```python
from build123d import *

# Parameters (mm, degrees)
SKETCH1_W           = 243
SKETCH1_H           = 30
BOSS_EXTRUDE1_DEPTH = 70
SKETCH2_W           = 120
SKETCH2_H           = 10
CUT_EXTRUDE1_DEPTH  = 70
FILLET1_R           = 3
SKETCH3_R           = 3
CUT_EXTRUDE2_DEPTH  = 20
SKETCH4_R           = 11.000191916
SKETCH4_R_2         = 5.90738233
BOSS_EXTRUDE2_DEPTH = 39
SKETCH5_R           = 1.5
CUT_EXTRUDE3_DEPTH  = 20


with BuildPart() as part:
    # Sketch1 → Boss-Extrude1 (new body)
    with BuildSketch(Plane(origin=(0, 0, 0), x_dir=(1, 0, 0), z_dir=(0, 1, 0))):
        with Locations((-94.428984733, -7.936828819)):
            Rectangle(SKETCH1_W, SKETCH1_H)
    extrude(amount=BOSS_EXTRUDE1_DEPTH)

    # Sketch2 → Cut-Extrude1 (cut)
    with BuildSketch(Plane(origin=(0, 70, 0), x_dir=(1, 0, 0), z_dir=(0, 1, 0))):
        with Locations((-45.928984733, 2.063171181)):
            Rectangle(SKETCH2_W, SKETCH2_H)
    extrude(amount=-CUT_EXTRUDE1_DEPTH, mode=Mode.SUBTRACT)

    # Fillet1
    fillet1_edges = [part.edges().sort_by_distance(p)[0] for p in [
        (14.071015267, 35, -7.063171181),
        (14.071015267, 35, 2.936828819),
        (-105.928984733, 35, 2.936828819),
        (-105.928984733, 35, -7.063171181),
    ]]
    fillet(fillet1_edges, radius=FILLET1_R)

    # Sketch3 → Cut-Extrude2 (cut)
    with BuildSketch(Plane(origin=(0, 0, 0), x_dir=(-1, 0, 0), z_dir=(0, -1, 0))):
        with Locations(Location((51.298984733, -12.077870123, 0), (0, 0, 90))):
            Circle(SKETCH3_R)
        with Locations(Location((185.928984733, -2.936828819, 0), (0, 0, 90))):
            Circle(SKETCH3_R)
    extrude(amount=-CUT_EXTRUDE2_DEPTH, mode=Mode.SUBTRACT)

    # Sketch4 → Boss-Extrude2 (add)
    with BuildSketch(Plane(origin=(0, 0, 0), x_dir=(-1, 0, 0), z_dir=(0, -1, 0))):
        with Locations((188.57546064, -9.351449297)):
            Circle(SKETCH4_R)
        with Locations((51.298984733, -12.077870123)):
            Circle(SKETCH4_R_2)
    extrude(amount=-BOSS_EXTRUDE2_DEPTH)

    # Sketch5 → Cut-Extrude3 (cut)
    with BuildSketch(Plane(origin=(0, 0, 0), x_dir=(-1, 0, 0), z_dir=(0, -1, 0))):
        with Locations(Location((51.298984733, -12.936828819, 0), (0, 0, 90))):
            Circle(SKETCH5_R)
        with Locations(Location((185.928984733, -2.936828819, 0), (0, 0, 90))):
            Circle(SKETCH5_R)
    extrude(amount=-CUT_EXTRUDE3_DEPTH, mode=Mode.SUBTRACT)


solid = part.part
```
Work out the finished part from the listing and answer in its coordinate system (mm). A direction names the side the tool comes from. Coordinates: 2 decimals unless noted, no trailing zeros. Loops run counter-clockwise (first coordinate to the right, second up) from the corner with the lowest first, then second, coordinate; pieces in that order, holes last. Notation, with made-up numbers: (-9.5, 15.25) -> (12.5, 15.25) arc R18 ccw to (12.5, 45.25) -> close; hole circle Ø2 at (31, -30.5). An arc over 180 degrees is marked (long way). Answer as CSV lines item,"result".
Q1. The part is cut by section B-B on x = -11.5. Write down the section's boundary in (y, z), and give its area (3 significant figures).
Findings:
outline,"(0, 2.94) -> (70, 2.94) -> (70, 22.94) -> (0, 22.94) -> close"
area,"1,400 mm²"
Q2. A tool of negligible diameter and unlimited length cuts with its end or side. For faces 5 (the face through (14.071, 35, -2)), 6 (the face through (-96, 35, 22.937)), from which of +Z, -Z, +X, -X, +Y, -Y can it reach the whole face along a straight path? Write none if from no direction.
Findings:
face 5,"-Z, +Y, -Y"
face 6,"+Z, +X, -X, +Y, -Y"
Q3. The part is cut by section A-A on y = 54.5. Write down the section's boundary in (x, z), and give its area (3 significant figures).
Findings:
outline,"(-215.93, -7.06) -> (-108.93, -7.06) arc R3 ccw to (-105.93, -4.06) -> (-105.93, -0.06) arc R3 cw to (-102.93, 2.94) -> (11.07, 2.94) arc R3 cw to (14.07, -0.06) -> (14.07, -4.06) arc R3 ccw to (17.07, -7.06) -> (27.07, -7.06) -> (27.07, 22.94) -> (-215.93, 22.94) -> close"
area,"6,090 mm²"
Q4. For a pull along X with two mould halves and no side action, classify faces 1 (the face through (22, 35, -7.063)), 2 (the face through (-105.929, 35, -2)), 3 (the face through (27.071, 35, 8)), 4 (the face through (-215.929, 35, 8)) as +X half, -X half, draft (parallel to the pull), parting line (faces both ways), or undercut.
Findings:
face 1,"draft"
face 2,"undercut"
face 3,"+X half"
face 4,"-X half"
Q5. Find the intervals of material crossed by probe 1 along Z at (x, y) = (3.5, 32); probe 2 along X at (y, z) = (33.5, -4.5); probe 3 along X at (y, z) = (34, 1.75), in increasing order.
Findings:
probe 1,"z = 2.94 to 22.94"
probe 2,"x = -215.93 to -105.96, 14.1 to 27.07"
probe 3,"x = -215.93 to -105.32, 13.46 to 27.07"
Q6. Each of these flat-tipped pins is pushed along its axis until it touches: pin 1 (0.9 mm diameter, centred on x = -51.5, z = 12.5, fed in from -Y); pin 2 (8 mm diameter, centred on x = -0.5, y = 46, fed in from -Z). Where does it stop, or does it pass through?
Findings:
pin 1,"stops at y = 20"
pin 2,"stops at z = 2.94"
